from build123d import *

# Parameters (mm, degrees)
F0_R     = 11.1
F1_DEPTH = 7


with BuildPart() as f1:
    # F0 (on Top) → F1 (new body)
    with BuildSketch(Plane.XY):
        with BuildLine():
            ThreePointArc((-20.1820022707, -9.9415058496), (-15.3539348415, -9.091091221), (-10.8430645172, -7.1713284596))
            ThreePointArc((-10.8430645172, -7.1713284596), (0.5582056386, -12.9880101041), (11.4183705824, -6.2145646061))
            ThreePointArc((11.4183705824, -6.2145646061), (16.4281860721, -1.651791194), (23, 0))
            ThreePointArc((23, 0), (24.7165507362, -1.0092828133), (24.6691871434, -3))
            ThreePointArc((24.6691871434, -3), (23.6178456633, -5.9816728989), (20.7402704139, -7.2913495265))
            ThreePointArc((20.7402704139, -7.2913495265), (18.8416140451, -10.5123262229), (15.2804029597, -11.6513444364))
            add(Edge.make_bspline(
                [(15.1405816519, -13.0223987218), (15.2788713972, -12.2898082007), (15.2804029597, -11.6513444364)],
                knots=[5.0540557872, 5.0540557872, 5.0540557872, 5.4022551178, 5.4022551178, 5.4022551178], degree=2, weights=[1, 0.9848828954, 1]))
            add(Edge.make_bspline(
                [(15.1405816519, -13.0223987218), (15.7602589992, -13.627545907), (16.4485412205, -14.1319848698)],
                knots=[2.4227067274, 2.4227067274, 2.4227067274, 2.5604830279, 2.5604830279, 2.5604830279], degree=2, weights=[1, 0.9976281496, 1]))
            ThreePointArc((16.4485412205, -14.1319848698), (16.7059454387, -14.0965620619), (16.7578368283, -14.3511578014))
            ThreePointArc((16.7578368283, -14.3511578014), (17.1960707743, -15.3819952285), (17.9098490626, -16.2452422082))
            ThreePointArc((17.9098490626, -16.2452422082), (20.2370224114, -15.5077337484), (22.6750224829, -15.3819952285))
            ThreePointArc((22.6750224829, -15.3819952285), (23.4818826617, -15.7752677938), (24.2466118351, -16.2452422082))
            ThreePointArc((24.2466118351, -16.2452422082), (25.3881728474, -15.9967588485), (26.3896299553, -15.3951034771))
            ThreePointArc((26.3896299553, -15.3951034771), (27.1373975838, -15.3951361034), (27.8500681048, -15.1687356707))
            ThreePointArc((27.8500681048, -15.1687356707), (30.0171813338, -15.3741600066), (32.0121236145, -16.2452422082))
            ThreePointArc((32.0121236145, -16.2452422082), (32.0780721748, -14.2146599803), (31.5934991398, -12.2416413867))
            ThreePointArc((31.5934991398, -12.2416413867), (32.8180555594, -11.9786425212), (33.9920036495, -11.5421190858))
            ThreePointArc((33.9920036495, -11.5421190858), (32.9938729979, -11.0530795037), (32.0121236145, -10.5319339782))
            ThreePointArc((32.0121236145, -10.5319339782), (33.1937729386, -8.8658671292), (34.7588080404, -7.5533356057))
            ThreePointArc((34.7588080404, -7.5533356057), (33.6044737815, -7.2274734783), (32.4501395226, -7.5533356057))
            ThreePointArc((32.4501395226, -7.5533356057), (33.4243691341, -1.2097485956), (32.4501395226, 5.1338384145))
            ThreePointArc((32.4501395226, 5.1338384145), (26.9985929856, 9.2793222728), (20.1820022707, 9.9415058496))
            ThreePointArc((20.1820022707, 9.9415058496), (15.3539348415, 9.091091221), (10.8430645172, 7.1713284596))
            ThreePointArc((10.8430645172, 7.1713284596), (-0.5582056386, 12.9880101041), (-11.4183705824, 6.2145646061))
            ThreePointArc((-11.4183705824, 6.2145646061), (-16.4281860721, 1.651791194), (-23, 0))
            ThreePointArc((-23, 0), (-24.7165507362, 1.0092828133), (-24.6691871434, 3))
            ThreePointArc((-24.6691871434, 3), (-23.6178456633, 5.9816728989), (-20.7402704139, 7.2913495265))
            ThreePointArc((-20.7402704139, 7.2913495265), (-18.8775642358, 10.4833581386), (-15.3726424061, 11.6555851871))
            add(Edge.make_bspline(
                [(-15.2804029597, 11.6513444364), (-15.325524504, 11.6549876637), (-15.3726424061, 11.6555851871)],
                knots=[0.2580425601, 0.2580425601, 0.2580425601, 0.2952358655, 0.2952358655, 0.2952358655], degree=2, weights=[1, 0.9998270872, 1]))
            add(Edge.make_bspline(
                [(-15.1405816519, 13.0223987218), (-15.2788713972, 12.2898082007), (-15.2804029597, 11.6513444364)],
                knots=[5.0540557872, 5.0540557872, 5.0540557872, 5.4022551178, 5.4022551178, 5.4022551178], degree=2, weights=[1, 0.9848828954, 1]))
            add(Edge.make_bspline(
                [(-15.1405816519, 13.0223987218), (-15.7602589992, 13.627545907), (-16.4485412205, 14.1319848698)],
                knots=[2.4227067274, 2.4227067274, 2.4227067274, 2.5604830279, 2.5604830279, 2.5604830279], degree=2, weights=[1, 0.9976281496, 1]))
            ThreePointArc((-16.4485412205, 14.1319848698), (-18.4202217975, 13.4084166875), (-20.5199281941, 13.3603723279))
            ThreePointArc((-20.5199281941, 13.3603723279), (-18.985312905, 14.5805065249), (-17.1960707743, 15.3819952285))
            ThreePointArc((-17.1960707743, 15.3819952285), (-17.5217288035, 15.8394422571), (-17.9098490626, 16.2452422082))
            ThreePointArc((-17.9098490626, 16.2452422082), (-20.2370224114, 15.5077337484), (-22.6750224829, 15.3819952285))
            ThreePointArc((-22.6750224829, 15.3819952285), (-23.4818826617, 15.7752677938), (-24.2466118351, 16.2452422082))
            ThreePointArc((-24.2466118351, 16.2452422082), (-25.3881728474, 15.9967588485), (-26.3896299553, 15.3951034771))
            ThreePointArc((-26.3896299553, 15.3951034771), (-27.1352445397, 15.395468841), (-27.8461648315, 15.1706720867))
            ThreePointArc((-27.8461648315, 15.1706720867), (-27.8481169003, 15.1697047499), (-27.8500681048, 15.1687356707))
            ThreePointArc((-27.8500681048, 15.1687356707), (-30.0171813338, 15.3741600066), (-32.0121236145, 16.2452422082))
            ThreePointArc((-32.0121236145, 16.2452422082), (-32.0780721748, 14.2146599803), (-31.5934991398, 12.2416413867))
            ThreePointArc((-31.5934991398, 12.2416413867), (-32.8180555594, 11.9786425212), (-33.9920036495, 11.5421190858))
            ThreePointArc((-33.9920036495, 11.5421190858), (-32.9938729979, 11.0530795037), (-32.0121236145, 10.5319339782))
            ThreePointArc((-32.0121236145, 10.5319339782), (-33.1937729386, 8.8658671292), (-34.7588080404, 7.5533356057))
            ThreePointArc((-34.7588080404, 7.5533356057), (-33.6044737815, 7.2274734783), (-32.4501395226, 7.5533356057))
            ThreePointArc((-32.4501395226, 7.5533356057), (-33.4243691341, 1.2097485956), (-32.4501395226, -5.1338384145))
            ThreePointArc((-32.4501395226, -5.1338384145), (-26.9985929856, -9.2793222728), (-20.1820022707, -9.9415058496))
        make_face()
        Circle(F0_R, mode=Mode.SUBTRACT)
        with BuildLine():
            ThreePointArc((-15.3726424061, 11.6555851871), (-15.326513354, 11.6536677218), (-15.2804029597, 11.6513444364))
            add(Edge.make_bspline(
                [(-15.2804029597, 11.6513444364), (-15.325524504, 11.6549876637), (-15.3726424061, 11.6555851871)],
                knots=[0.2580425601, 0.2580425601, 0.2580425601, 0.2952358655, 0.2952358655, 0.2952358655], degree=2, weights=[1, 0.9998270872, 1]))
        make_face()
    extrude(amount=F1_DEPTH)


solid = f1.part
CAD build for the part. Positions are in the model's coordinates, mm. A direction names the side the tool comes from. Give positions to 0.01 mm unless a question says otherwise; leave off trailing zeros. Order: outer loops, then holes, each group sorted by start corner. A loop starts at its lowest first (then second) coordinate and runs counter-clockwise, first axis right, second up. Notation, with made-up numbers: (-24.5, 75.5) - (26.5, 75.5) arc R20 ccw to (26.5, 83.5) - close; hole circle Ø11 at (13.25, 85.5). An arc over 180 degrees is marked (long way). Answer in a Markdown table with one row per item.
1. Probe probe 1 along Y at (x, z) = (0, 4.5); probe 2 along Y at (x, z) = (10, 3.5); probe 3 along Y at (x, z) = (-12, 2.25). List the from-to ranges inside material, lowest first. Write a range as [from, to].
Data:
| item | result |
|---|---|
| probe 1 | y = [-13, -11.1], [11.1, 13] |
| probe 2 | y = [-8.31, -4.82], [4.82, 8.31] |
| probe 3 | y = [-7.78, 5.4] |
2. Saw through at A-A, the plane x = 0. Give the cut face in (y, z).
Data:
| item | result |
|---|---|
| outline | (-13, 0) - (-11.1, 0) - (-11.1, 7) - (-13, 7) - close; (11.1, 0) - (13, 0) - (13, 7) - (11.1, 7) - close |
3. Tool access for faces 4 (the cylindrical face through (33.01, -11.06, 3.45)), 5 (the cylindrical face through (25.373, -16.003, 3.451)), 6 (the cylindrical face through (-23.648, 5.948, 3.451)), 7 (the cylindrical face through (17.19, -15.37, 3.45)): list every direction of +Z, -Z, +X, -X, +Y, -Y with a clear straight run to the whole face (end or side of a thin tool).
Data:
| item | result |
|---|---|
| face 4 | +Z, -Z, +X |
| face 5 | +Z, -Z, -Y |
| face 6 | +Z, -Z |
| face 7 | +Z, -Z, -X, -Y |
4. Pull direction Y, two halves, no side cores. Call faces 1 (the cylindrical face through (20.203, -15.514, 3.451)), 2 (the flat face through (7.2, -10.6, 7)), 3 (the cylindrical face through (18.88, -10.48, 3.45)): pulls with the +Y half, pulls with the -Y half, needs draft (parallel to the pull), parting line crosses it, or undercut.
Data:
| item | result |
|---|---|
| face 1 | pulls with the -Y half |
| face 2 | needs draft |
| face 3 | undercut |
5. Saw through at B-B, the plane x = 7. Give the cut face in (y, z), plus the area to 3 significant figures.
Data:
| item | result |
|---|---|
| outline | (-10.95, 0) - (-8.61, 0) - (-8.61, 7) - (-10.95, 7) - close; (8.61, 0) - (10.95, 0) - (10.95, 7) - (8.61, 7) - close |
| area | 32.8 mm² |
6. Saw through at C-C, the plane x = -13.5. Give the cut face in (y, z), plus the area to 3 significant figures.
Data:
| item | result |
|---|---|
| outline | (-8.45, 0) - (3.75, 0) - (3.75, 7) - (-8.45, 7) - close |
| area | 85.4 mm² |
7. Flat gauge pins, fed straight in: pin 1 (1.5 mm diameter, centred on x = 1, z = 3.5, fed in from -Y); pin 2 (2 mm diameter, centred on y = -2, z = 4, fed in from +X); pin 3 (1 mm diameter, centred on x = -4.5, z = 3.5, fed in from -Y). Where does each tip first touch, or does it go through?
Data:
| item | result |
|---|---|
| pin 1 | stops at y = -13 |
| pin 2 | stops at x = 33.42 |
| pin 3 | stops at y = -12.37 |
